Answer from the drawing. Dimensions are ordinates in mm from the lowest x, y and z of the part. Round coordinates to 2 decimals unless told otherwise and drop trailing zeros. Loops run counter-clockwise (first coordinate to the right, second up) from the corner with the lowest first, then second, coordinate; pieces in that order, holes last. Notation, with made-up numbers: M 73.25,15 L 132.25,15 A31 ccw 132.25,46 Z; hole C 71,34 d10. An arc over 180 degrees is marked long. Write each question's results on one line, items separated by ' | '.
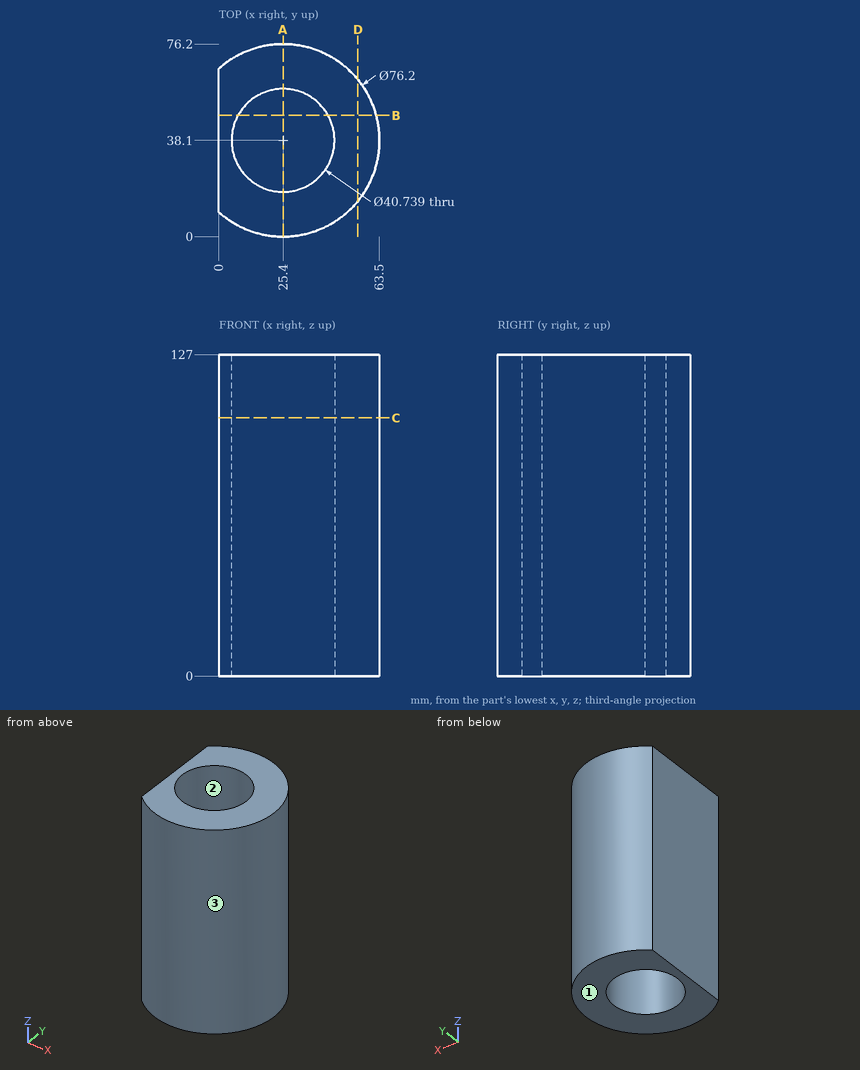
1. Find section A-A, the plane x = 25.4. Give the vertices of the cut face in (y, z), then the cut area to 3 significant figures.
Completed:
outline: M 0,0 L 17.73,0 L 17.73,127 L 0,127 Z; M 58.47,0 L 76.2,0 L 76.2,127 L 58.47,127 Z | area: 4,500 mm2
2. Determine the mould class of the marked faces 1, 2 and 3 for opening direction X: released by +X, released by -X, zero draft, split by the parting line, or undercut.
Completed:
face 1: zero draft | face 2: undercut | face 3: split by the parting line
3. Given P1, Ø1.5, axis at x = 18, z = 48.5, coming from the +Y side (1 decimal); P2, Ø6, axis at x = 37.5, y = 29, coming from the +Z side; P3, Ø6, axis at x = 25.5, z = 17.5, coming from the +Y side; P4, Ø5, axis at y = 12.5, z = 38.5, coming from the +X side, each flat-ended and moving along its own axis, determine where each tip first touches the part or whether it passes through.
Completed:
P1: stops at y = 75.6 | P2: passes through | P3: stops at y = 76.2 | P4: stops at x = 55.7
4. Find the intervals of material crossed by L1, parallel to X at y = 39, z = 65.5; L2, parallel to Y at x = 25, z = 35 (1 decimal); L3, parallel to X at y = 38, z = 51, in increasing order.
Completed:
L1: x = 0 to 5.05, 45.75 to 63.49 | L2: y = 0 to 17.7, 58.5 to 76.2 | L3: x = 0 to 5.03, 45.77 to 63.5
5. Find section B-B, the plane y = 48. Give the vertices of the cut face in (x, z), then the cut area to 3 significant figures.
Completed:
outline: M 0,0 L 7.6,0 L 7.6,127 L 0,127 Z; M 43.2,0 L 62.19,0 L 62.19,127 L 43.2,127 Z | area: 3,380 mm2
6. Find section C-C, the plane z = 102. Give the vertices of the cut face in (x, y).
Completed:
outline: M 0,9.7 A38.1 ccw long 0,66.5 Z; hole C 25.4,38.1 d40.74
7. Find section D-D, the plane x = 55. Give the vertices of the cut face in (y, z), then the cut area to 3 significant figures.
Completed:
outline: M 14.11,0 L 62.09,0 L 62.09,127 L 14.11,127 Z | area: 6,090 mm2
